Design review of the part built by this model. Coordinates are the model's own, in mm. A direction names the side the tool comes from. Round coordinates to 2 decimals unless told otherwise and drop trailing zeros. Write each loop counter-clockwise with the first axis right and the second up, starting at its lowest first coordinate (ties: lowest second). Pieces come first, ordered by that corner, then holes. Notation, with made-up numbers: M 28.25,-30.75 L 57.25,-30.75 A10 cw 57.25,-14.75 Z; hole C 49,-33 d5. An arc over 180 degrees is marked long. One line per question, with ' | ' between items. Start each with the question number.
Item 1: Insertion check: pin 1 Ø1 at (x, y) = (-1, -3.5) entering from -Z; pin 2 Ø1.5 at (x, z) = (-1.5, -2.5) entering from -Y; pin 3 Ø0.6 at (x, z) = (-1, 0) entering from +Y. Each pin has a flat end and moves straight along its axis. Give the tip position at first contact, or say it passes through.
Item 2: For L1, parallel to Y at x = 0, z = -2.75; L2, parallel to Y at x = -1, z = -2.25; L3, parallel to X at y = -4, z = -0.25, list the stretches that pass through material, from the lowest coordinate up.
Item 3: Machinability: for faces 1 (the face through (0, -12, 0)), 2 (the face through (-1.5, -5.79, -0.07)), 3 (the face through (0.05, 1.51, -0.58)), which of the approach directions +Z, -Z, +X, -X, +Y, -Y give a long, thin tool a straight path to every point of the face, cutting with its end or side? Answer none if there is none.
Item 4: Add section C-C, the plane y = -10.75. State the section outline as (x, z) points.
Item 5: Add section A-A, the plane x = 0. State the section outline as (y, z) points, and give its area (3 significant figures).
Item 6: Add section B-B, the plane z = 0. State the section outline as (x, y) points, and give its area (3 significant figures).
Autodesk Inventor part; units mm, degrees
ref_plane "工作平面1" through (3.5, 0, 0) normal (1, 0, 0) x (0, 1, 0)
ref_plane "XZ Plane" through (0, 0, 0) normal (0, 1, 0) x (-1, 0, 0)
ref_plane "XY Plane" through (0, 0, 0) normal (0, 0, 1) x (1, 0, 0)
sketch "草图1" plane through (0, 0, 0) normal (0, 0, 1) x (1, 0, 0)
  line L0 (-3.5, 2) -> (0, 2)
  line L1 (0, 2) -> (0, 0)
  line L2 (0, 0) -> (-1.5, 0)
  line L3 (-1.5, 0) -> (-3.5, 2)
  line L4 (0, -0.4) -> (0, 2.4)
  dimension "d0" = 3.5
  dimension "d1" = 2
  dimension "d2" = 1.5
revolve "旋转1" add sketch "草图1" angle 360 about axis through (0, -10, 0) along (0, 1, 0)
sketch "草图2" plane through (0, 0, 0) normal (0, -1, 0) x (1, 0, 0)
  circle A0 centre (0, 0) radius 1.5
  dimension "d4" = 3
extrude "拉伸1" add sketch "草图2" along normal blind 12
chamfer "倒角1" distance 0.25 angle 45 1 edges at (-1.5, -12, 0)
thread "螺纹1"
ref_plane "工作平面1" through (3.5, 0, 0) normal (1, 0, 0) x (0, 1, 0)
sketch "草图3" plane through (3.5, 0, 0) normal (1, 0, 0) x (0, 1, 0)
  line L0 (2, -0.75) -> (1, -0.4)
  line L1 (1, -0.4) -> (1, 0.4)
  line L2 (2, -3.5) -> (2, 3.5)
  line L3 (1, 0.4) -> (2, 0.75)
  line L4 (2, 0.75) -> (2, -0.75)
  point P0 (0, 0)
  point P1 (2, 0)
  dimension "d13" = 1
  dimension "d14" = 0.8
  dimension "d15" = 1.5
extrude "拉伸2" cut sketch "草图3" against normal blind 7
properties part number "载板连接销固定螺丝"
Computed values:
1) pin 1: stops at z = -1.41 | pin 2: stops at y = 0.67 | pin 3: stops at y = 1
2) L1: y = 1.25 to 2 | L2: y = 0.96 to 2 | L3: x = -1.48 to 1.48
3) face 1: +Z, -Z, +X, -X, -Y | face 2: -Y | face 3: +X, -X, +Y
4) outline: C 0,0 d3
5) outline: M -12,-1.25 L -11.75,-1.5 L 0,-1.5 L 2,-3.5 L 2,-0.75 L 1,-0.4 L 1,0.4 L 2,0.75 L 2,3.5 L 0,1.5 L -11.75,1.5 L -12,1.25 Z | area: 44.8 mm^2
6) outline: M -2.5,1 L -1.5,0 L -1.5,-11.75 L -1.25,-12 L 1.25,-12 L 1.5,-11.75 L 1.5,0 L 2.5,1 Z | area: 39.9 mm^2
